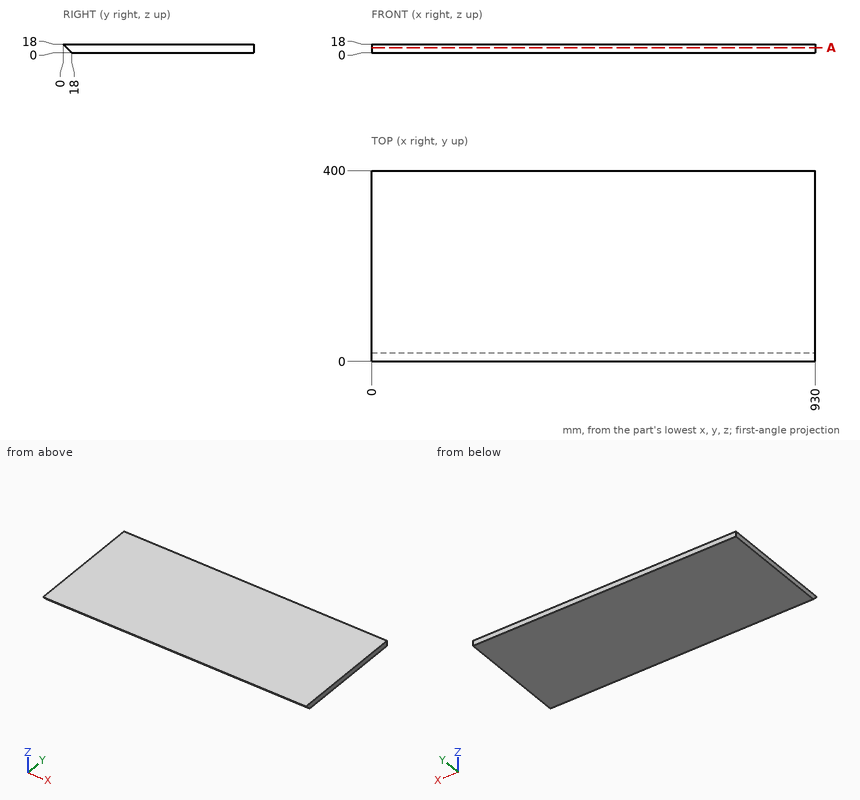
Geometry: see drawing. Coordinates: mm, zero at the bounding-box minimum. Give positions to 0.01 mm unless a question says otherwise; leave off trailing zeros. Order: outer loops, then holes, each group sorted by start corner. A loop starts at its lowest first (then second) coordinate and runs counter-clockwise, first axis right, second up.
1. Line query: probe 1 along Y at (x, z) = (280, 17.25); probe 2 along Y at (x, z) = (241.5, 11). Output: solid intervals per line, ascending.
Computed:
probe 1: y = 0.75 to 400
probe 2: y = 7 to 400
2. Cut plane A-A (z = 10.5). Return loops of the section in (x, y), and give its area (3 significant figures).
Computed:
outline: (0, 7.5) - (930, 7.5) - (930, 400) - (0, 400) - close
area: 365,000 mm2
3. Pin query (flat end, axial travel): pin 1 Ø1.5 at (x, z) = (794, 11) entering from -Y. Return the tip coordinate at first contact, or that it passes through.
Computed:
pin 1: stops at y = 6.25
